```python
from build123d import *

# Parameters (mm, degrees)
F0_W     = 100
F0_H     = 200
F2_R     = 50
F3_DEPTH = 200
F5_DEPTH = 50


with BuildPart() as f1:
    # F0 (on Front) → F1 (revolve)
    with BuildSketch(Plane.XZ):
        with Locations((-50, 0)):
            Rectangle(F0_W, F0_H)
    revolve(axis=Axis((0, 0, 0), (0, 0, 1)))

    # F2 (on face) → F3 (cut)
    with BuildSketch(Plane(origin=(0, 0, -100), x_dir=(1, 0, 0), z_dir=(0, 0, -1))):
        Circle(F2_R)
    extrude(amount=-F3_DEPTH, mode=Mode.SUBTRACT)

    # F4 (on face) → F5 (join)
    with BuildSketch(Plane(origin=(0, 0, -100), x_dir=(1, 0, 0), z_dir=(0, 0, -1))):
        with BuildLine():
            ThreePointArc((-96.875, 24.803919), (-100, 0), (-96.875, -24.803919))
            ThreePointArc((-96.875, -24.803919), (-81.25, -16.535946), (-75, 0))
            ThreePointArc((-75, 0), (-81.25, 16.535946), (-96.875, 24.803919))
        make_face()
        with BuildLine():
            ThreePointArc((-96.875, 24.803919), (-125, 0), (-96.875, -24.803919))
            ThreePointArc((-96.875, -24.803919), (-100, 0), (-96.875, 24.803919))
        make_face()
        with BuildLine():
            ThreePointArc((-24.803919, -96.875), (-1.565573, -124.950931), (25, -100))
            ThreePointArc((25, -100), (24.950931, -98.434427), (24.803919, -96.875))
            ThreePointArc((24.803919, -96.875), (0, -100), (-24.803919, -96.875))
        make_face()
        with BuildLine():
            ThreePointArc((-24.803919, -96.875), (0, -100), (24.803919, -96.875))
            ThreePointArc((24.803919, -96.875), (0, -75), (-24.803919, -96.875))
        make_face()
        with BuildLine():
            ThreePointArc((-24.803919, 96.875), (0, 100), (24.803919, 96.875))
            ThreePointArc((24.803919, 96.875), (24.950931, 98.434427), (25, 100))
            ThreePointArc((25, 100), (-1.565573, 124.950931), (-24.803919, 96.875))
        make_face()
        with BuildLine():
            ThreePointArc((-24.803919, 96.875), (0, 75), (24.803919, 96.875))
            ThreePointArc((24.803919, 96.875), (0, 100), (-24.803919, 96.875))
        make_face()
        with BuildLine():
            ThreePointArc((100, 0), (99.215674, -12.5), (96.875, -24.803919))
            ThreePointArc((96.875, -24.803919), (116.535946, -18.75), (125, 0))
            ThreePointArc((125, 0), (116.535946, 18.75), (96.875, 24.803919))
            ThreePointArc((96.875, 24.803919), (99.215674, 12.5), (100, 0))
        make_face()
        with BuildLine():
            ThreePointArc((96.875, 24.803919), (75, 0), (96.875, -24.803919))
            ThreePointArc((96.875, -24.803919), (99.215674, -12.5), (100, 0))
            ThreePointArc((100, 0), (99.215674, 12.5), (96.875, 24.803919))
        make_face()
    extrude(amount=F5_DEPTH)

    # F6: F1 across plane


with BuildPart() as f1_1:
    add(f1.part)
    add(f1.part.mirror(Plane.XY))


solid = f1_1.part
```
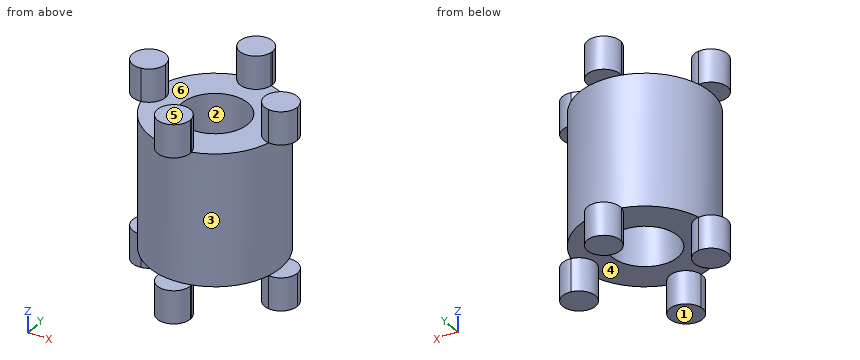
The model under review builds one solid part; all positions refer to its coordinate system, in mm. Face numbers are marked on the shaded views. A direction names the side the tool comes from. Round coordinates to 2 decimals unless told otherwise and drop trailing zeros. Write each loop counter-clockwise with the first axis right and the second up, starting at its lowest first coordinate (ties: lowest second). Pieces come first, ordered by that corner, then holes. Notation, with made-up numbers: (34.5, 42) - (46.5, 42) arc R22 ccw to (46.5, 77) - close; hole circle Ø4 at (-12, 18.25). An arc over 180 degrees is marked (long way). Answer as CSV lines item,"result". Start each with the question number.
(1) We need section D-D on y = 87. State the section outline as (x, z) points.
(2) To check wall thickness, follow line 1 (Z direction, x = 15.5, y = 101); line 2 (Y direction, x = 0, z = 33). State the ranges of each line that lie inside material, in increasing order.
(3) For the marked faces 5 and 6, list the 3-axis set-ups (+Z, -Z, +X, -X, +Y, -Y) from which the entire face can be reached by the end or side of a thin tool; tool diameter is ignored.
(4) We need section A-A on x = 0. State the section outline as (y, z) points.
(5) We need section C-C on z = 61. State the section outline as (x, y) points, plus the area to 3 significant figures.
(6) Draft analysis for pull direction Y (two halves, no side actions). For the marked faces 1, 2, 3 and 4, state which applies: pulls with the +Y half, pulls with the -Y half, needs draft (parallel to the pull), parting line crosses it, or undercut.
(7) We need section B-B on y = -34. State the section outline as (x, z) points.
(8) For pin 1 Ø8 at (x, z) = (-56, 19.5) entering from -Y; pin 2 Ø12 at (x, z) = (64, -36) entering from -Y; pin 3 Ø2 at (x, y) = (-76.5, -53) entering from +Z, all flat-tipped, find the tip position at first contact; note any pin that passes through.
Worked answers:
1,outline,"(-49.31, -100) - (-21.35, -100) - (-21.35, -150) - (21.35, -150) - (21.35, -100) - (49.31, -100) - (49.31, 100) - (21.35, 100) - (21.35, 150) - (-21.35, 150) - (-21.35, 100) - (-49.31, 100) - close"
2,line 1,"-150 to -100, 100 to 150"
2,line 2,"-100 to -50, 50 to 100"
3,face 5,"+Z, +X, -X, +Y, -Y"
3,face 6,"+Z"
4,outline,"(-125, -150) - (-75, -150) - (-75, -100) - (-50, -100) - (-50, 100) - (-75, 100) - (-75, 150) - (-125, 150) - (-125, 100) - (-100, 100) - (-100, -100) - (-125, -100) - close; (50, -100) - (75, -100) - (75, -150) - (125, -150) - (125, -100) - (100, -100) - (100, 100) - (125, 100) - (125, 150) - (75, 150) - (75, 100) - (50, 100) - close"
5,outline,"circle Ø200 at (0, 0); hole circle Ø100 at (0, 0)"
5,area,"23,600 mm²"
6,face 1,"needs draft"
6,face 2,"undercut"
6,face 3,"parting line crosses it"
6,face 4,"undercut"
7,outline,"(-94.04, -100) - (-36.66, -100) - (-36.66, 100) - (-94.04, 100) - close; (36.66, -100) - (94.04, -100) - (94.04, 100) - (36.66, 100) - close"
8,pin 1,"y = -85.42"
8,pin 2,"y = -81.46"
8,pin 3,"z = 100"
